Could you check a few things on this drawing? It's one solid part, dimensions in mm from its lowest x, y, z. Round coordinates to 2 decimals unless told otherwise and drop trailing zeros. Write each loop counter-clockwise with the first axis right and the second up, starting at its lowest first coordinate (ties: lowest second). Pieces come first, ordered by that corner, then holes. Notation, with made-up numbers: (45.5, -33.75) -> (95.5, -33.75) arc R29 cw to (95.5, -6.75) -> close; hole circle Ø8 at (-14, 74.25). An arc over 180 degrees is marked (long way). Answer as CSV lines item,"result".
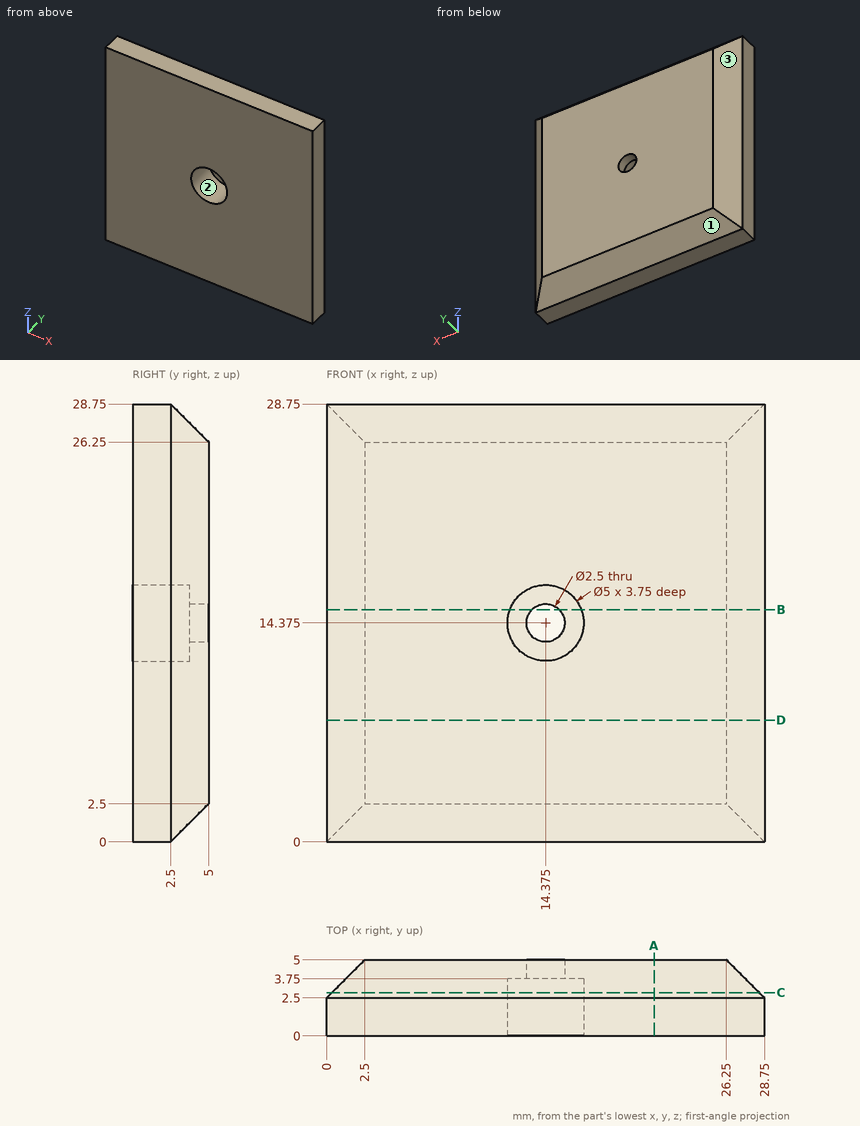
1. Suppose I cut it at B-B on z = 15.25. Please give me the cut outline in (x, y), and give its area (3 significant figures).
Numbers:
outline,"(0, 0) -> (12.03, 0) -> (12.03, 3.75) -> (13.48, 3.75) -> (13.48, 5) -> (2.5, 5) -> (0, 2.5) -> close; (15.27, 3.75) -> (16.72, 3.75) -> (16.72, 0) -> (28.75, 0) -> (28.75, 2.5) -> (26.25, 5) -> (15.27, 5) -> close"
area,"118 mm^2"
2. Suppose I cut it at D-D on z = 8. Please give me the cut outline in (x, y), and give its area (4 significant figures).
Numbers:
outline,"(0, 0) -> (28.75, 0) -> (28.75, 2.5) -> (26.25, 5) -> (2.5, 5) -> (0, 2.5) -> close"
area,"137.5 mm^2"
3. For pin 1 Ø3 at (x, z) = (14.375, 14.375) entering from -Y, with a flat end and sliding along its axis, tell me the tip position at first contact or that it passes through.
Numbers:
pin 1,"stops at y = 3.75"
4. Suppose I cut it at C-C on y = 2.85. Please give me the cut outline in (x, z) (3 decimals), and give its area (3 significant figures).
Numbers:
outline,"(0.35, 0.35) -> (28.4, 0.35) -> (28.4, 28.4) -> (0.35, 28.4) -> close; hole circle Ø5 at (14.375, 14.375)"
area,"767 mm^2"
5. If I drill on line 1 (Z direction, x = 15.25, y = 1.1); line 2 (X direction, y = 4.3, z = 7); line 3 (X direction, y = 3, z = 13.75), over which ranges is the centre line in solid material (lowest first)?
Numbers:
line 1,"z = 0 to 12.03, 16.72 to 28.75"
line 2,"x = 1.8 to 26.95"
line 3,"x = 0.5 to 11.95, 16.8 to 28.25"
6. If we mould it in two halves opening along Z, with no side actions, what happens to the marked faces 1, 2 and 3? For each: released by +Z, released by -Z, zero draft, split by the parting line, or undercut.
Numbers:
face 1,"released by -Z"
face 2,"undercut"
face 3,"zero draft"
7. Suppose I cut it at A-A on x = 21.5. Please give me the cut outline in (y, z).
Numbers:
outline,"(0, 0) -> (2.5, 0) -> (5, 2.5) -> (5, 26.25) -> (2.5, 28.75) -> (0, 28.75) -> close"
